Can you work these out from the model? Positions are in its coordinate system, mm. Face numbers are marked on the shaded views. A direction names the side the tool comes from. Give positions to 0.01 mm unless a question says otherwise; leave off trailing zeros. Write each loop counter-clockwise with the first axis right and the second up, starting at its lowest first coordinate (ties: lowest second). Pieces come first, ordered by that corner, then holes.
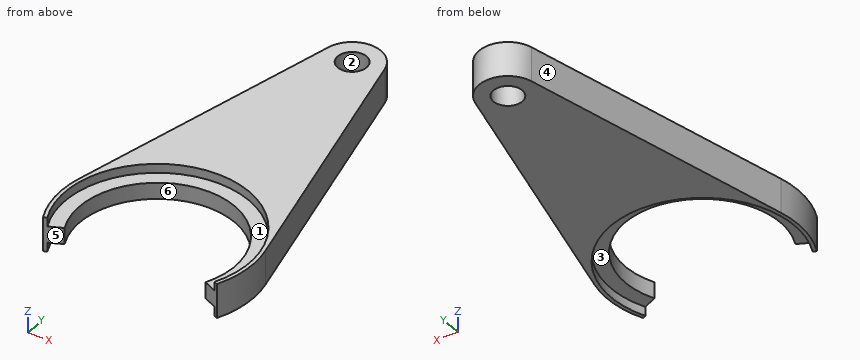
Autodesk Inventor part; units mm, degrees
ref_plane "Work Plane1" through (0, 0, 2.25) normal (0, 0, 1) x (1, 0, 0)
ref_plane "YZ Plane" through (0, 0, 0) normal (1, 0, 0) x (0, 1, 0)
ref_plane "XZ Plane" through (0, 0, 0) normal (0, 1, 0) x (-1, 0, 0)
sketch "Sketch1" plane through (0, 0, 0) normal (0, 0, 1) x (1, 0, 0)
  circle A0 centre (0, 0) radius 21.5
  arc A1 (-25.7817, 6.1281) -> (25.7817, 6.1281) centre (0, 0) ccw
  line L0 (0, 0) -> (0, 80) construction
  circle A2 centre (0, 80) radius 4
  arc A3 (7.7832, 81.85) -> (-7.7832, 81.85) centre (0, 80) ccw
  line L1 (-7.7832, 81.85) -> (-25.7817, 6.1281)
  line L2 (7.7832, 81.85) -> (25.7817, 6.1281)
  dimension "d0" = 43
  dimension "d1" = 8
  dimension "d2" = 80
  dimension "d3" = 8
  dimension "d4" = 5
extrude "Extrusion1" add sketch "Sketch1" along normal blind 4.5
sketch "Sketch2" plane through (0, 0, 4.5) normal (0, 0, 1) x (1, 0, 0)
  circle A0 centre (0, 0) radius 21.5
  circle A1 centre (0, 80) radius 4
  arc A2 (-25.7817, 6.1281) -> (25.7817, 6.1281) centre (0, 0) ccw
  line L0 (25.7817, 6.1281) -> (7.7832, 81.85)
  arc A3 (7.7832, 81.85) -> (-7.7832, 81.85) centre (0, 80) ccw
  line L1 (-7.7832, 81.85) -> (-25.7817, 6.1281)
  circle A4 centre (0, 0) radius 25.5
  dimension "d7" = 51
extrude "Extrusion2" add sketch "Sketch2" along normal blind 2.5 contours L1 A3 L0 A2
ref_plane "Work Plane1" through (0, 0, 2.25) normal (0, 0, 1) x (1, 0, 0)
mirror "Mirror1" about plane through (0, 0, 2.25) normal (0, 0, 1) of "Extrusion2"
sketch "Sketch3" plane through (0, 0, 7) normal (0, 0, 1) x (1, 0, 0)
  arc A0 (-25.7817, 6.1281) -> (25.7817, 6.1281) centre (0, 0) ccw construction
  line L0 (0, 0) -> (-24.0172, -11.1994)
  line L1 (0, 0) -> (24.0172, -11.1994)
  arc A1 (-24.0172, -11.1994) -> (24.0172, -11.1994) centre (0, 0) ccw
  line L2 (0, 0) -> (0, -26.5) construction
  dimension "d10" = 130
extrude "Extrusion3" cut sketch "Sketch3" against normal through all
properties part number "fork"
1) Please list where these lines run through material, in increasing order: L1, parallel to X at y = 0, z = 5; L2, parallel to Z at x = -9, y = 23.5; L3, parallel to X at y = 15, z = 1.5.
Values follow:
L1: x = -26.5 to -25.5, 25.5 to 26.5
L2: z = 0 to 4.5
L3: x = -23.67 to -15.4, 15.4 to 23.67
2) For the marked faces 1, 2 and 3, which set-ups out of +Z, -Z, +X, -X, +Y, -Y let a thin tool reach every point of the face, with its end or its side?
Values follow:
face 1: +Z
face 2: +Z, -Z
face 3: -Z
3) Suppose I cut it at C-C on z = 3.5. Write out the boundary of the cut face in (x, y), plus the area to 3 significant figures.
Values follow:
outline: (-25.78, 6.13) arc R26.5 ccw to (-24.02, -11.2) - (-19.49, -9.09) arc R21.5 cw (long way) to (19.49, -9.09) - (24.02, -11.2) arc R26.5 ccw to (25.78, 6.13) - (7.78, 81.85) arc R8 ccw to (-7.78, 81.85) - close; hole circle Ø8 at (0, 80)
area: 2,260 mm2
4) For pin 1 Ø1.5 at (x, z) = (6, 5) entering from -Y; pin 2 Ø3 at (x, z) = (7, -1) entering from -Y; pin 3 Ø2 at (y, z) = (72.5, 0.5) entering from -X, each with a flat end and sliding along its axis, tell me the tip position at first contact or that it passes through.
Values follow:
pin 1: stops at y = 20.48
pin 2: stops at y = 19.91
pin 3: stops at x = -10.24
5) Suppose I cut it at A-A on y = 0. Write out the boundary of the cut face in (x, z).
Values follow:
outline: (-26.5, -2.5) - (-25.5, -2.5) - (-25.5, 0) - (-21.5, 0) - (-21.5, 4.5) - (-25.5, 4.5) - (-25.5, 7) - (-26.5, 7) - close; (21.5, 0) - (25.5, 0) - (25.5, -2.5) - (26.5, -2.5) - (26.5, 7) - (25.5, 7) - (25.5, 4.5) - (21.5, 4.5) - close
6) Suppose I cut it at D-D on x = -20.5. Write out the boundary of the cut face in (y, z), plus the area to 3 significant figures.
Values follow:
outline: (-9.56, 0) - (-6.48, 0) - (-6.48, 4.5) - (-9.56, 4.5) - close; (6.48, 0) - (15.17, 0) - (15.17, -2.5) - (28.35, -2.5) - (28.35, 7) - (15.17, 7) - (15.17, 4.5) - (6.48, 4.5) - close
area: 178 mm2
7) If we mould it in two halves opening along Y, with no side actions, what happens to the marked faces 4, 5 and 6? For each: +Y half, -Y half, draft (parallel to the pull), parting line (faces both ways), or undercut.
Values follow:
face 4: +Y half
face 5: -Y half
face 6: undercut
8) Suppose I cut it at B-B on x = 0. Write out the boundary of the cut face in (y, z), plus the area to 3 significant figures.
Values follow:
outline: (21.5, 0) - (25.5, 0) - (25.5, -2.5) - (76, -2.5) - (76, 7) - (25.5, 7) - (25.5, 4.5) - (21.5, 4.5) - close; (84, -2.5) - (88, -2.5) - (88, 7) - (84, 7) - close
area: 536 mm2
